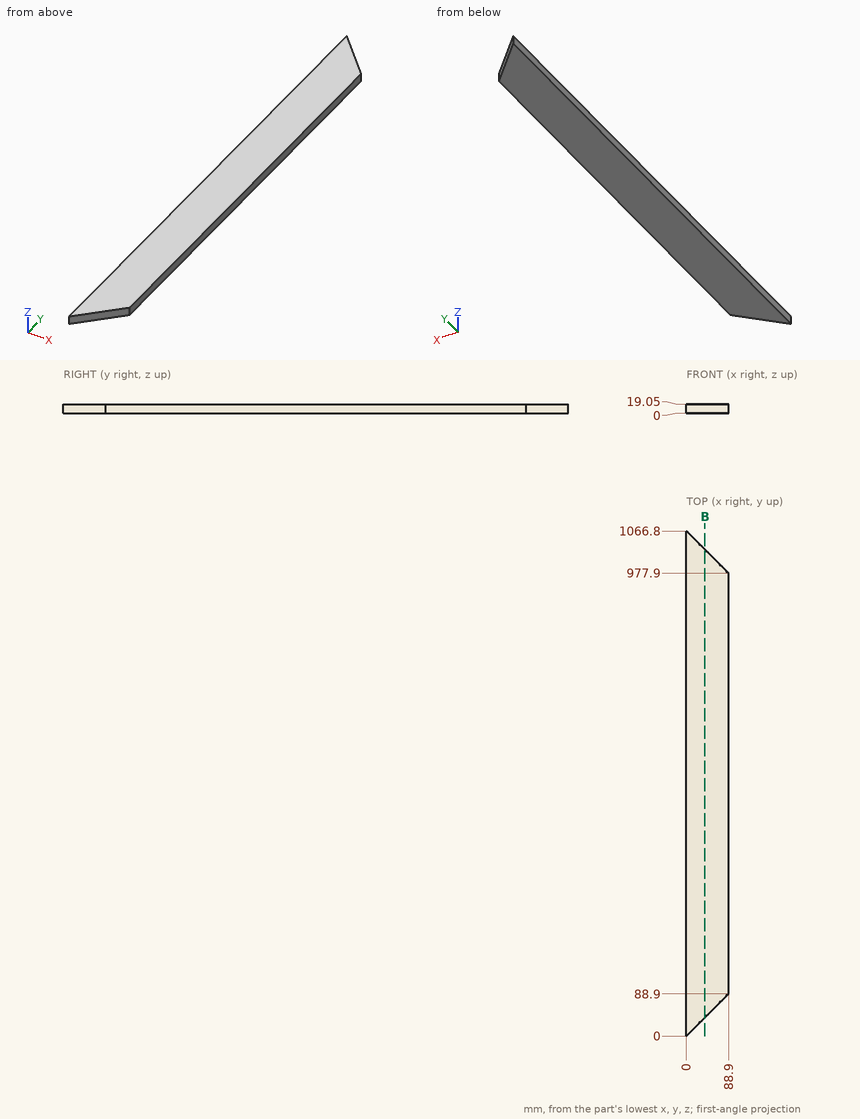
Source: three-view drawing plus pictorial views. Frame: mm from the lowest corner of the part. Give positions to 0.01 mm unless a question says otherwise; leave off trailing zeros. Loops run counter-clockwise (first coordinate to the right, second up) from the corner with the lowest first, then second, coordinate; pieces in that order, holes last.
1) Line query: L1, parallel to Y at x = 56.5, z = 16.5; L2, parallel to Y at x = 37, z = 14.75; L3, parallel to X at y = 1003.5, z = 1.25. Output: solid intervals per line, ascending.
A:
L1: y = 56.5 to 1010.3
L2: y = 37 to 1029.8
L3: x = 0 to 63.3
2) Section query B-B on x = 39. Return the cut outline in (y, z), and give its area (3 significant figures).
A:
outline: (39, 0) - (1027.8, 0) - (1027.8, 19.05) - (39, 19.05) - close
area: 18,800 mm2
3) Contact query for flat-ended pins moving along their axis: pin 1 (1.5 mm diameter, centred on x = 49, z = 6, fed in from +Y); pin 2 (3 mm diameter, centred on x = 34, z = 3.5, fed in from -Y). Output: stop coordinate, or through.
A:
pin 1: stops at y = 1018.55
pin 2: stops at y = 32.5
